The model under review builds one solid part; all positions refer to its coordinate system, in mm. A direction names the side the tool comes from. Round coordinates to 2 decimals unless told otherwise and drop trailing zeros. Order: outer loops, then holes, each group sorted by start corner. A loop starts at its lowest first (then second) coordinate and runs counter-clockwise, first axis right, second up. Notation, with made-up numbers: (-27.75, 69.5) -> (-14.75, 69.5) arc R11 ccw to (-14.75, 88.5) -> close; hole circle Ø5 at (30, 36.5). An arc over 180 degrees is marked (long way). Use a Markdown table: item, result. Add a question column.
```python
from build123d import *

# Parameters (mm, degrees)
F0_R      = 24.8798987062
F1_DEPTH  = 60
F1_FACE_R = 24.8798987062
F2_ANGLE  = 180


with BuildPart() as f1:
    # F0 (on Front) → F1 (new body, symmetric)
    with BuildSketch(Plane.XZ):
        Polygon((-42.4695287796, 7.1159532226), (-27.3973606527, -33.2217141986), (15.0721681269, -40.3376674212), (42.4695287796, -7.1159532226), (27.3973606527, 33.2217141986), (-15.0721681269, 40.3376674212), align=None)
        Circle(F0_R, mode=Mode.SUBTRACT)
    extrude(amount=F1_DEPTH, both=True)

    # F1_face (on face) → F2 (revolve)
    with BuildSketch(Plane(origin=(0, 60, 0), x_dir=(1, 0, 0), z_dir=(0, 1, 0))):
        Polygon((-42.4695287796, -7.1159532226), (-15.0721681269, -40.3376674212), (27.3973606527, -33.2217141986), (42.4695287796, 7.1159532226), (15.0721681269, 40.3376674212), (-27.3973606527, 33.2217141986), align=None)
        Circle(F1_FACE_R, mode=Mode.SUBTRACT)
    revolve(axis=Axis((6.1625962629, 60, 36.7796908099), (0.9862515905, 0, -0.1652507194)), revolution_arc=F2_ANGLE)


solid = f1.part
```
Q1. To check wall thickness, follow line 1 along Y through (x, z) = (17.5, -24); line 2 along Y through (x, z) = (22.5, 44); line 3 along Z through (x, y) = (0, -7). State the ranges of each line that lie inside material, in increasing order.
Q2. Add section A-A, the plane y = -45.5. Give the boundary of the cut face in (x, z), then the cut area to 3 significant figures.
Q3. Draft analysis for pull direction Z (two halves, no side actions). For faces 1 (the face through (-35.42, 99.09, 42.87)), 2 (the face through (35.04, -0.84, 12.77)), 3 (the face through (-5.39, 0.84, -24.29)), 4 (the face through (-23.233, 74.238, 41.388)), state which applies: released by +Z, released by -Z, zero draft, split by the parting line, or undercut.
Q4. For faces 5 (the face through (-28.58, -0.84, 23.96)), 6 (the face through (-35.04, -0.84, -12.77)), 7 (the face through (6.46, -0.84, 36.73)), list the 3-axis set-ups (+Z, -Z, +X, -X, +Y, -Y) from which the entire face can be reached by the end or side of a thin tool; tool diameter is ignored.
Q5. For pin 1 (1.5 mm diameter, centred on x = 42, y = 59.5, fed in from -Z); pin 2 (5 mm diameter, centred on y = 83.5, z = 88.5, fed in from -X); pin 3 (8 mm diameter, centred on x = 22, y = 73, fed in from -Z); pin 4 (10 mm diameter, centred on y = 53.5, z = 55.5, fed in from -X), all flat-tipped, find the tip position at first contact; note any pin that passes through.
Return value:
| question | item | result |
|---|---|---|
| 1 | line 1 | -60 to 106.8 |
| 1 | line 2 | 60 to 74.34, 116.35 to 133.94 |
| 1 | line 3 | -37.81 to -24.88, 24.88 to 37.81 |
| 2 | outline | (-42.47, 7.12) -> (-27.4, -33.22) -> (15.07, -40.34) -> (42.47, -7.12) -> (27.4, 33.22) -> (-15.07, 40.34) -> close; hole circle Ø49.76 at (0, 0) |
| 2 | area | 2,870 mm² |
| 3 | face 1 | split by the parting line |
| 3 | face 2 | released by +Z |
| 3 | face 3 | undercut |
| 3 | face 4 | undercut |
| 4 | face 5 | +Z, -X, -Y |
| 4 | face 6 | -Z, -X, +Y, -Y |
| 4 | face 7 | +Z, +X, -Y |
| 5 | pin 1 | z = -8.59 |
| 5 | pin 2 | x = -22.08 |
| 5 | pin 3 | z = -35.88 |
| 5 | pin 4 | through |
